from build123d import *

# Parameters (mm, degrees)
SKETCH1_W                                           = 90
SKETCH1_H                                           = 45
BOSS_EXTRUDE1_DEPTH                                 = 30
SKETCH2_W                                           = 5
SKETCH2_H                                           = 45
BOSS_EXTRUDE2_DEPTH                                 = 8
CBORE_START                                         = 5
CBORE_SLOT_FOR_M6_HEX_SOCKET_HEAD_CAP_SC_DEPTH      = 25
CBORE_SLOT_FOR_M6_HEX_SOCKET_HEAD_CA_3_DEPTH        = 5
CHAMFER2_SIZE                                       = 4
CBORE_FOR_M3_HEX_SOCKET_HEAD_CAP_SCREW1_D           = 3.4
CBORE_FOR_M3_HEX_SOCKET_HEAD_CAP_SCREW1_DEPTH       = 5
CBORE_FOR_M3_HEX_SOCKET_HEAD_CAP_SCREW1_CBORE_D     = 6.5
CBORE_FOR_M3_HEX_SOCKET_HEAD_CAP_SCREW1_CBORE_DEPTH = 3.5
CBORE_FOR_M3_HEX_SOCKET_HEAD_CAP_SCREW2_D           = 3.4
CBORE_FOR_M3_HEX_SOCKET_HEAD_CAP_SCREW2_CBORE_D     = 6.5
CBORE_FOR_M3_HEX_SOCKET_HEAD_CAP_SCREW2_CBORE_DEPTH = 3.5
CUT_EXTRUDE1_REACH                                  = 86.977
SKETCH11_W                                          = 12
SKETCH11_H                                          = 2.5
FILLET1_R                                           = 2
CUT_EXTRUDE3_DEPTH                                  = 17.5


# Read off the part's stored shape, not the designer's step: CBORE SLOT for M6 Hex Socket Head Cap Screw1
with BuildPart() as part:
    # Sketch1 → Boss-Extrude1 (new body)
    with BuildSketch(Plane(origin=(0, 0, 0), x_dir=(1, 0, 0), z_dir=(0, 1, 0))):
        Rectangle(SKETCH1_W, SKETCH1_H)
    extrude(amount=BOSS_EXTRUDE1_DEPTH)

    # Sketch2 → Boss-Extrude2 (add)
    with BuildSketch(Plane(origin=(0, 30, 0), x_dir=(1, 0, 0), z_dir=(0, 1, 0))):
        with Locations((-25.1, 0)):
            Rectangle(SKETCH2_W, SKETCH2_H)
        with Locations((25.1, 0)):
            Rectangle(SKETCH2_W, SKETCH2_H)
    extrude(amount=BOSS_EXTRUDE2_DEPTH)

    # CBORE SLOT for M6 Hex Socket Head Ca 2 → CBORE SLOT for M6 Hex Socket Head Cap Screw1 (cut)
    with BuildSketch(Plane(origin=(0, 0, 0), x_dir=(1, 0, 0), z_dir=(0, 1, 0)).offset(CBORE_START)):
        with BuildLine():
            Line((-5.5, 14.2), (-5.5, -14.2))
            ThreePointArc((-5.5, -14.2), (0, -19.7), (5.5, -14.2))
            Line((5.5, -14.2), (5.5, 14.2))
            ThreePointArc((5.5, 14.2), (0, 19.7), (-5.5, 14.2))
        make_face()
        with BuildLine():
            Line((32, 14.2), (32, -14.2))
            ThreePointArc((32, -14.2), (37.5, -19.7), (43, -14.2))
            Line((43, -14.2), (43, 14.2))
            ThreePointArc((43, 14.2), (37.5, 19.7), (32, 14.2))
        make_face()
        with BuildLine():
            Line((-43, 14.2), (-43, -14.2))
            ThreePointArc((-43, -14.2), (-37.5, -19.7), (-32, -14.2))
            Line((-32, -14.2), (-32, 14.2))
            ThreePointArc((-32, 14.2), (-37.5, 19.7), (-43, 14.2))
        make_face()
    extrude(amount=CBORE_SLOT_FOR_M6_HEX_SOCKET_HEAD_CAP_SC_DEPTH, mode=Mode.SUBTRACT)

    # CBORE SLOT for M6 Hex Socket Head Ca 3 o → CBORE SLOT for M6 Hex Socket Head Ca 3 (cut)
    with BuildSketch(Plane(origin=(0, 0, 0), x_dir=(1, 0, 0), z_dir=(0, 1, 0))):
        with BuildLine():
            Line((-3.3, 14.2), (-3.3, -14.2))
            ThreePointArc((-3.3, -14.2), (0, -17.5), (3.3, -14.2))
            Line((3.3, -14.2), (3.3, 14.2))
            ThreePointArc((3.3, 14.2), (0, 17.5), (-3.3, 14.2))
        make_face()
        with BuildLine():
            Line((34.2, 14.2), (34.2, -14.2))
            ThreePointArc((34.2, -14.2), (37.5, -17.5), (40.8, -14.2))
            Line((40.8, -14.2), (40.8, 14.2))
            ThreePointArc((40.8, 14.2), (37.5, 17.5), (34.2, 14.2))
        make_face()
        with BuildLine():
            Line((-40.8, 14.2), (-40.8, -14.2))
            ThreePointArc((-40.8, -14.2), (-37.5, -17.5), (-34.2, -14.2))
            Line((-34.2, -14.2), (-34.2, 14.2))
            ThreePointArc((-34.2, 14.2), (-37.5, 17.5), (-40.8, 14.2))
        make_face()
    extrude(amount=CBORE_SLOT_FOR_M6_HEX_SOCKET_HEAD_CA_3_DEPTH, mode=Mode.SUBTRACT)

    # Chamfer2
    chamfer2_edges = [part.edges().sort_by_distance(p)[0] for p in [
        (-45, 15, -22.5),
        (45, 15, -22.5),
        (45, 15, 22.5),
        (-45, 15, 22.5),
    ]]
    chamfer(chamfer2_edges, length=CHAMFER2_SIZE)

    # CBORE for M3 Hex Socket Head Cap Screw1
    with Locations(Plane(origin=(27.6, 0, 0), x_dir=(0, 0, -1), z_dir=(1, 0, 0))):
        with Locations((-10, 34), (10, 34)):
            CounterBoreHole(CBORE_FOR_M3_HEX_SOCKET_HEAD_CAP_SCREW1_D / 2, CBORE_FOR_M3_HEX_SOCKET_HEAD_CAP_SCREW1_CBORE_D / 2, CBORE_FOR_M3_HEX_SOCKET_HEAD_CAP_SCREW1_CBORE_DEPTH, depth=CBORE_FOR_M3_HEX_SOCKET_HEAD_CAP_SCREW1_DEPTH)

    # CBORE for M3 Hex Socket Head Cap Screw2 (through all)
    with Locations(Plane.ZY.offset(27.6)):
        with Locations((-10, 34), (10, 34)):
            CounterBoreHole(CBORE_FOR_M3_HEX_SOCKET_HEAD_CAP_SCREW2_D / 2, CBORE_FOR_M3_HEX_SOCKET_HEAD_CAP_SCREW2_CBORE_D / 2, CBORE_FOR_M3_HEX_SOCKET_HEAD_CAP_SCREW2_CBORE_DEPTH)

    # Cut-Extrude1: up to this face of the body (flat: up to its plane)
    cut_extrude1_end = Plane(part.part.faces().sort_by_distance((-27.6, 34, 0))[0])
    # Sketch11 → Cut-Extrude1 (cut, up to the picked face)
    with BuildSketch(Plane(origin=(27.6, 0, 0), x_dir=(0, 0, -1), z_dir=(1, 0, 0)), mode=Mode.PRIVATE) as cut_extrude1_sk1:
        with Locations((0, 36.75)):
            Rectangle(SKETCH11_W, SKETCH11_H)
    cut_extrude1_tool1 = split(extrude(cut_extrude1_sk1.sketch, amount=-CUT_EXTRUDE1_REACH, mode=Mode.PRIVATE), bisect_by=cut_extrude1_end, keep=Keep.BOTH, mode=Mode.PRIVATE)
    add(cut_extrude1_tool1.solids().sort_by(Axis((27.6, 36.75, 0), (-1, 0, 0)))[0], mode=Mode.SUBTRACT)

    # Fillet1
    fillet1_edges = [part.edges().sort_by_distance(p)[0] for p in [
        (-25.1, 35.5, -6),
        (25.1, 35.5, -6),
        (-25.1, 35.5, 6),
        (25.1, 35.5, 6),
    ]]
    fillet(fillet1_edges, radius=FILLET1_R)

    # Sketch13 → Cut-Extrude3 (cut)
    with BuildSketch(Plane(origin=(0, 30, 0), x_dir=(1, 0, 0), z_dir=(0, 1, 0))):
        Polygon((-45, 18.5), (-45, -18.5), (-41, -22.5), (-27.6, -22.5), (-27.6, 22.5), (-41, 22.5), align=None)
        Polygon((45, -18.5), (45, 18.5), (41, 22.5), (27.6, 22.5), (27.6, -22.5), (41, -22.5), align=None)
    extrude(amount=-CUT_EXTRUDE3_DEPTH, mode=Mode.SUBTRACT)


solid = part.part
Input: part model. Units: mm. Frame: model coordinates. A direction names the side the tool comes from. Coordinates: 2 decimals unless noted, no trailing zeros. Order: outer loops, then holes, each group sorted by start corner. A loop starts at its lowest first (then second) coordinate and runs counter-clockwise, first axis right, second up.
1. Cut plane D-D, the plane x = -37.5. Return loops of the section in (y, z).
Checked values:
outline: (0, -22.5) - (12.5, -22.5) - (12.5, -19.7) - (5, -19.7) - (5, -17.5) - (0, -17.5) - close; (0, 17.5) - (5, 17.5) - (5, 19.7) - (12.5, 19.7) - (12.5, 22.5) - (0, 22.5) - close
2. Ray query, line 1 along Z through (x, y) = (23, 34); line 2 along X through (y, z) = (9.5, -10); line 3 along X through (y, z) = (36, 18). Return the intervals inside material, ascending.
Checked values:
line 1: z = -22.5 to -11.7, -8.3 to 8.3, 11.7 to 22.5
line 2: x = -45 to -43, -32 to -5.5, 5.5 to 32, 43 to 45
line 3: x = -27.6 to -22.6, 22.6 to 27.6
3. Contact query for flat-ended pins moving along their axis: P1, Ø7.5, axis at y = 28.5, z = -1.5, coming from the -X side; P2, Ø6, axis at y = 34, z = -10, coming from the +X side; P3, Ø5.5, axis at x = 2.5, z = 5, coming from the +Y side. Output: stop coordinate, or through.
Checked values:
P1: stops at x = -27.6
P2: stops at x = 24.1
P3: stops at y = 5
4. Access query for faces 4 (the cylindrical face through (25.06, 36.1, -5.43)), 5 (the flat face through (34, 5, 0)), 6 (the flat face through (22.6, 34, 0)), 7 (the cylindrical face through (0.1, 2.5, -17.5)), 8 (the flat face through (-31, 12.5, 0)). Directions: +Z, -Z, +X, -X, +Y, -Y. A direction counts if a zero-diameter tool reaches every point of the face in a straight line with its end or side. Return the directions, or none.
Checked values:
face 4: +X, -X, +Y
face 5: +Y
face 6: +Z, -Z, +Y
face 7: +Y, -Y
face 8: +Z, -Z, -X, +Y
5. Cut plane C-C, the plane y = 34. Count the separate pieces of the cut face and the enclosed holes in it, plus the area to 3 significant figures.
Checked values:
separate pieces: 6
enclosed holes: 0
area: 339 mm2
6. Cut plane B-B, the plane x = 0. Return loops of the section in (y, z), plus the area to 3 significant figures.
Checked values:
outline: (0, -22.5) - (30, -22.5) - (30, -19.7) - (5, -19.7) - (5, -17.5) - (0, -17.5) - close; (0, 17.5) - (5, 17.5) - (5, 19.7) - (30, 19.7) - (30, 22.5) - (0, 22.5) - close
area: 190 mm2
7. Draft query along X for faces 1 (the flat face through (-25, 38, -14)), 2 (the flat face through (-43, 9, 0)), 3 (the flat face through (24.1, 32.6, 8.6)). Return one class per face: +X half, -X half, draft (parallel to the pull), parting line (faces both ways), or undercut.
Checked values:
face 1: draft
face 2: undercut
face 3: +X half
8. Cut plane A-A, the plane y = 14. Return loops of the section in (x, z), plus the area to 3 significant figures.
Checked values:
outline: (-27.6, -22.5) - (27.6, -22.5) - (27.6, 22.5) - (-27.6, 22.5) - close; hole (-5.5, -14.2) arc R5.5 ccw to (5.5, -14.2) - (5.5, 14.2) arc R5.5 ccw to (-5.5, 14.2) - close
area: 2,080 mm2
